```python
from build123d import *

# Parameters (mm, degrees)
F0_W     = 90
F0_H     = 20
F1_DEPTH = 25
F2_R     = 5
F3_DEPTH = 15
F4_R     = 4
F5_DEPTH = 25.001
F6_R     = 5
F7_R     = 3
F8_R     = 3
F9_R     = 2
F10_R    = 2


with BuildPart() as f1:
    # F0 (on Top) → F1 (new body)
    with BuildSketch(Plane.XY):
        with Locations((45, 10)):
            Rectangle(F0_W, F0_H)
    extrude(amount=-F1_DEPTH)

    # F2 (on Top) → F3 (join)
    with BuildSketch(Plane.XY):
        with Locations((10, 10)):
            Circle(F2_R)
        with Locations((80, 10)):
            Circle(F2_R)
    extrude(amount=F3_DEPTH)

    # F4 (on Top) → F5 (cut, through all)
    with BuildSketch(Plane.XY):
        with Locations((45, 10)):
            Circle(F4_R)
    extrude(amount=-F5_DEPTH, mode=Mode.SUBTRACT)

    # F6
    f6_edges = [f1.edges().sort_by_distance(p)[0] for p in [
        (0, 0, -12.5),
        (0, 20, -12.5),
        (90, 0, -12.5),
        (90, 20, -12.5),
    ]]
    fillet(f6_edges, radius=F6_R)

    # F7
    f7_edges = [f1.edges().sort_by_distance(p)[0] for p in [
        (5, 10, 15),
        (75, 10, 15),
    ]]
    fillet(f7_edges, radius=F7_R)

    # F8
    f8_edges = [f1.edges().sort_by_distance(p)[0] for p in [
        (41, 10, -25),
    ]]
    fillet(f8_edges, radius=F8_R)

    # F9
    f9_edges = [f1.edges().sort_by_distance(p)[0] for p in [
        (45, 0, -25),
    ]]
    fillet(f9_edges, radius=F9_R)

    # F10
    f10_edges = [f1.edges().sort_by_distance(p)[0] for p in [
        (45, 0, 0),
    ]]
    fillet(f10_edges, radius=F10_R)


solid = f1.part
```
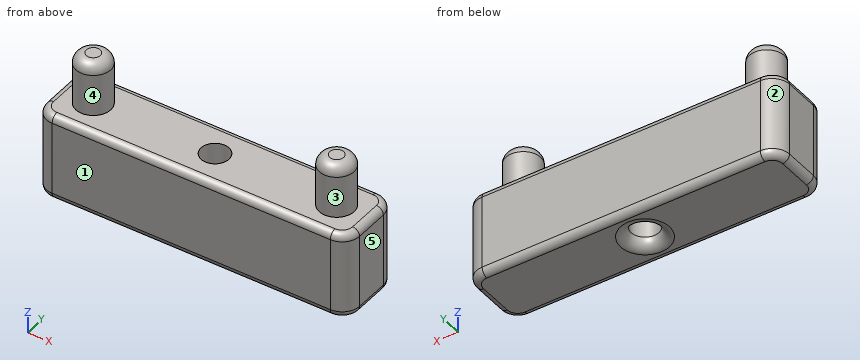
Part model, mm, in its own coordinate system. Face numbers are marked on the shaded views. A direction names the side the tool comes from. Round coordinates to 2 decimals unless told otherwise and drop trailing zeros. Order: outer loops, then holes, each group sorted by start corner. A loop starts at its lowest first (then second) coordinate and runs counter-clockwise, first axis right, second up. Notation, with made-up numbers: M 38.25,69 L 47.25,69 A10 cw 47.25,86 Z; hole C 75,-23.5 d3. An arc over 180 degrees is marked long. Put each result on its own line as item: value. Start each with the question number.
1. Slice it at B-B on z = -20. List the corners of the cut face in (x, y).
2. Drill centre lines: probe 1 along Y at (x, z) = (45, -10); probe 2 along Z at (x, y) = (37, 4); probe 3 along X at (y, z) = (10.75, -17.5). Where is each one in solid material? Low to high. Write a range as [from, to].
3. Tool access for the marked faces 4 and 5: list every direction of +Z, -Z, +X, -X, +Y, -Y with a clear straight run to the whole face (end or side of a thin tool).
4. Slice it at D-D on z = 7. List the corners of the cut face in (x, y).
5. Slice it at A-A on x = 45. List the corners of the cut face in (y, z).
6. Slice it at C-C on x = 60.5. List the corners of the cut face in (y, z).
7. Drop flat-ended pins along their axis: pin 1 (1.5 mm diameter, centred on y = 5.5, z = -0.5, fed in from +X); pin 2 (5 mm diameter, centred on x = 25.5, y = 11, fed in from +Z); pin 3 (7 mm diameter, centred on x = 45, y = 10, fed in from -Z); pin 4 (5 mm diameter, centred on y = 14, z = 10, fed in from -X). Give the stop position or say it passes through.
8. Two-plate mould, pull along X, no slides. Class the marked faces 1, 2 and 3: +X half, -X half, draft (parallel to the pull), parting line (faces both ways), or undercut.
Findings:
1. outline: M 0,5 A5 ccw 5,0 L 85,0 A5 ccw 90,5 L 90,15 A5 ccw 85,20 L 5,20 A5 ccw 0,15 Z; hole C 45,10 d8
2. probe 1: [0, 6], [14, 20]
2. probe 2: [-25, 0]
2. probe 3: [0, 41.07], [48.93, 90]
3. face 4: +Z
3. face 5: +Z, -Z, +X, +Y, -Y
4. outline: C 10,10 d10; C 80,10 d10
5. outline: M 0,-23 A2 ccw 2,-25 L 3,-25 A3 ccw 6,-22 L 6,0 L 2,0 A2 ccw 0,-2 Z; M 14,-22 A3 ccw 17,-25 L 18,-25 A2 ccw 20,-23 L 20,-2 A2 ccw 18,0 L 14,0 Z
6. outline: M 0,-23 A2 ccw 2,-25 L 18,-25 A2 ccw 20,-23 L 20,-2 A2 ccw 18,0 L 2,0 A2 ccw 0,-2 Z
7. pin 1: x = 89.85
7. pin 2: z = 0
7. pin 3: through
7. pin 4: x = 5.23
8. face 1: draft
8. face 2: -X half
8. face 3: undercut
